Could you check a few things on this model? Use its own coordinates, in mm. Coordinates: 2 decimals unless noted, no trailing zeros. Order: outer loops, then holes, each group sorted by start corner. A loop starts at its lowest first (then second) coordinate and runs counter-clockwise, first axis right, second up. Notation, with made-up numbers: M -5.5,10 L 40.5,10 A20 ccw 40.5,15 Z; hole C 87,10.5 d1. An arc over 180 degrees is marked long. Write item = value, one per line. Start each with the question number.
from build123d import *

# Parameters (mm, degrees)
SKETCH2_R                        = 0.635
SKETCH2_R_2                      = 1.5875
BOSS_EXTRUDE1_DEPTH              = 1.5875
F_10_0_1935_DIAMETER_HOLE1_D     = 4.9149
BOSS_EXTRUDE2_START              = 1.5875
BOSS_EXTRUDE2_DEPTH              = 1.5875
F_10_32_TAPPED_HOLE1_D           = 4.0386
F_10_32_TAPPED_HOLE1_DEPTH       = 9.398
F_10_32_TAPPED_HOLE1_CSINK_D     = 5.3086
F_10_32_TAPPED_HOLE1_CSINK_ANGLE = 90
F_10_32_TAPPED_HOLE1_TIP         = 1.213317848
BOSS_EXTRUDE3_START              = -3.175
BOSS_EXTRUDE3_DEPTH              = 3.175
F_10_32_TAPPED_HOLE2_D           = 4.0386


with BuildPart() as part:
    # Sketch2 → Boss-Extrude1 (new body)
    with BuildSketch(Plane.XY.offset(-44.699989247)):
        with BuildLine():
            Line((-22.87049754, -6.312086997), (25.389436119, -6.392107131))
            ThreePointArc((25.389436119, -6.392107131), (31.749956355, -0.052644824), (25.410494049, 6.307875411))
            Line((25.410494049, 6.307875411), (-22.84943961, 6.387895545))
            ThreePointArc((-22.84943961, 6.387895545), (-29.209959846, 0.048433239), (-22.87049754, -6.312086997))
        make_face()
        with Locations((25.399965084, -0.04211586)):
            Circle(SKETCH2_R, mode=Mode.SUBTRACT)
        Circle(SKETCH2_R_2, mode=Mode.SUBTRACT)
        with Locations((-22.859968575, 0.037904274)):
            Circle(SKETCH2_R, mode=Mode.SUBTRACT)
    extrude(amount=BOSS_EXTRUDE1_DEPTH)

    # #10 (0.1935) Diameter Hole1 (through all)
    with Locations(Plane.XY.offset(-43.112489247)):
        with Locations((-22.859968575, 0.037904274)):
            Hole(F_10_0_1935_DIAMETER_HOLE1_D / 2)

    # Sketch5 → Boss-Extrude2 (add)
    with BuildSketch(Plane(origin=(0, 0, -44.699989247), x_dir=(-1, 0, 0), z_dir=(0, 0, -1)).offset(BOSS_EXTRUDE2_START)):
        with BuildLine():
            Line((-25.389436119, -6.392107131), (-17.769446594, -6.379472373))
            ThreePointArc((-17.769446594, -6.379472373), (-15.974631383, -5.632546579), (-15.233661671, -3.835264278))
            Line((-15.233661671, -3.835264278), (-15.246296429, 3.784725247))
            ThreePointArc((-15.246296429, 3.784725247), (-15.993222223, 5.579540457), (-17.790504524, 6.320510169))
            Line((-17.790504524, 6.320510169), (-25.410494049, 6.307875411))
            ThreePointArc((-25.410494049, 6.307875411), (-31.749956355, -0.052644824), (-25.389436119, -6.392107131))
        make_face()
    extrude(amount=-BOSS_EXTRUDE2_DEPTH)

    # #10-32 Tapped Hole1
    with Locations(Plane.XY.offset(-43.112489247)):
        with Locations((25.399965084, -0.04211586)):
            CounterSinkHole(F_10_32_TAPPED_HOLE1_D / 2, F_10_32_TAPPED_HOLE1_CSINK_D / 2, depth=F_10_32_TAPPED_HOLE1_DEPTH, counter_sink_angle=F_10_32_TAPPED_HOLE1_CSINK_ANGLE)
            with Locations((0, 0, -(F_10_32_TAPPED_HOLE1_DEPTH + F_10_32_TAPPED_HOLE1_TIP / 2))):  # 118° drill point
                Cone(0, F_10_32_TAPPED_HOLE1_D / 2, F_10_32_TAPPED_HOLE1_TIP, mode=Mode.SUBTRACT)

    # Sketch8 → Boss-Extrude3 (add)
    with BuildSketch(Plane.XY.offset(-43.112489247).offset(BOSS_EXTRUDE3_START)):
        with BuildLine():
            Line((28.055366234, 5.726015964), (40.639944134, -0.067385375))
            Line((40.639944134, -0.067385375), (28.036223326, -5.81902182))
            ThreePointArc((28.036223326, -5.81902182), (31.749956355, -0.052644824), (28.055366234, 5.726015964))
        make_face()
    extrude(amount=BOSS_EXTRUDE3_DEPTH)

    # #10-32 Tapped Hole2 (through all)
    with Locations(Plane.XY.offset(-43.112489247)):
        with Locations((0, 0)):
            Hole(F_10_32_TAPPED_HOLE2_D / 2)


solid = part.part
(1) Imagine slicing it at A-A on x = 0. List the corners of the cut face in (y, z) for me.
(2) Will these pins go through, and if not, where does the flat tip stop? P1, Ø6.5, axis at x = 0, y = 0, coming from the -Z side; P2, Ø1, axis at x = 30.5, z = -44.5, coming from the -Y side; P3, Ø2.5, axis at x = 25.4, y = -0.04, coming from the +Z side; P4, Ø1, axis at y = 1.5, z = -46, coming from the +X side.
(3) Imagine slicing it at D-D on x = -21.5. List the corners of the cut face in (y, z) for me.
(4) Thinking about a two-plate mould opening in Y: for faces 1 (the cylindrical face through (26.762, -6.244, -44.722)), 2 (the cylindrical face through (-25.204, 0.776, -43.917)), 3 (the cylindrical face through (15.974, 5.56, -45.505)), which applies, released by +Y, released by -Y, zero draft, split by the parting line, or undercut?
(5) Imagine slicing it at C-C on y = 1. Give the number of separate pieces and of enclosed holes in the cut face, plus the area to 3 significant figures.
(6) Imagine slicing it at B-B on z = -45.5. List the corners of the cut face in (x, y) for me, plus the area to 3 significant figures.
(7) Please list where these lines run through material, in increasing order: probe 1 along X at (y, z) = (-1.25, -44.1); probe 2 along Z at (x, y) = (14, 1.25); probe 3 along X at (y, z) = (-0.75, -45). Write a range as from..to.
Response:
q1.outline = M -6.35,-44.7 L -2.02,-44.7 L -2.02,-43.11 L -6.35,-43.11 Z; M 2.02,-44.7 L 6.35,-44.7 L 6.35,-43.11 L 2.02,-43.11 Z
q2.P1 = -44.7
q2.P2 = -4.92
q2.P3 = through
q2.P4 = 38.32
q3.outline = M -6.31,-44.7 L -2.01,-44.7 L -2.01,-43.11 L -6.31,-43.11 Z; M 2.08,-44.7 L 6.39,-44.7 L 6.39,-43.11 L 2.08,-43.11 Z
q4.face_1 = released by -Y
q4.face_2 = undercut
q4.face_3 = released by +Y
q5.separate_pieces = 4
q5.enclosed_holes = 0
q5.area = 120 mm2
q6.outline = M 15.23,-3.84 A2.54 ccw 17.77,-6.38 L 25.39,-6.39 A6.35 ccw 28.04,-5.82 L 40.64,-0.07 L 28.06,5.73 A6.35 ccw 25.41,6.31 L 17.79,6.32 A2.54 ccw 15.25,3.78 Z; hole C 25.4,-0.04 d4.04
q6.area = 219 mm2
q7.probe_1 = -29.08..-24.95, -20.77..-1.59, 1.59..23.78, 27.02..38.05
q7.probe_2 = -44.7..-43.11
q7.probe_3 = 15.24..23.51, 27.29..39.14
